Build history of the part. All positions in model axes, mm. A direction names the side the tool comes from. Round coordinates to 2 decimals unless told otherwise and drop trailing zeros. Loops run counter-clockwise (first coordinate to the right, second up) from the corner with the lowest first, then second, coordinate; pieces in that order, holes last. Notation, with made-up numbers: (79, 43) - (109, 43) arc R12 cw to (109, 61) - close; hole circle Ø6 at (-9, -5). An arc over 180 degrees is marked (long way). Use a Markdown table: item, result.
from build123d import *

# Parameters (mm, degrees)
SKETCH_1_W               = 56
SKETCH_1_H               = 14
F_56X14_3_3MM_DEPTH      = 3
SKETCH_2_W               = 40
SKETCH_2_H               = 11
CUT_EXTRUDE_40_4_3_DEPTH = 3
SKETCH_3_W               = 8
SKETCH_3_H               = 25
F_5_M2_5X10_DEPTH        = 5
SKETCH_4_R               = 1.55
CUT_EXTRUDE_3_1_48_DEPTH = 5
SKETCH_5_R               = 1.8
CUT_EXTRUDE_993_DEPTH    = 3


with BuildPart() as part:
    # 草图1 → 相机小底脚56x14_厚3_单向3mm (new body)
    with BuildSketch(Plane(origin=(0, 0, 0), x_dir=(1, 0, 0), z_dir=(0, 1, 0))):
        with Locations((0, 2)):
            Rectangle(SKETCH_1_W, SKETCH_1_H)
    extrude(amount=F_56X14_3_3MM_DEPTH)

    # 草图2 → 底脚中央40宽镂空_只留后横梁4_贯穿底脚3 (cut)
    with BuildSketch(Plane(origin=(0, 0, 0), x_dir=(1, 0, 0), z_dir=(0, 1, 0))):
        with Locations((0, -0.5)):
            Rectangle(SKETCH_2_W, SKETCH_2_H)
    extrude(amount=CUT_EXTRUDE_40_4_3_DEPTH, mode=Mode.SUBTRACT)

    # 草图3 → 双耳支撑臂厚5_沿用M2.5x10尺寸链 (add)
    with BuildSketch(Plane.XY):
        with Locations((-24, 15.5)):
            Rectangle(SKETCH_3_W, SKETCH_3_H)
        with Locations((24, 15.5)):
            Rectangle(SKETCH_3_W, SKETCH_3_H)
    extrude(amount=F_5_M2_5X10_DEPTH)

    # 草图4 → 双耳原孔3.1_孔距48_圆孔不加大_贯穿 (cut)
    with BuildSketch(Plane.XY):
        with Locations((-24, 24)):
            Circle(SKETCH_4_R)
        with Locations((24, 24)):
            Circle(SKETCH_4_R)
    extrude(amount=CUT_EXTRUDE_3_1_48_DEPTH, mode=Mode.SUBTRACT)

    # 草图5 → Cut-Extrude 993 (cut)
    with BuildSketch(Plane(origin=(0, 0, 0), x_dir=(1, 0, 0), z_dir=(0, 1, 0))):
        with Locations(Location((-24, 4.5, 0), (0, 0, 270))):
            Circle(SKETCH_5_R)
        with Locations(Location((24, 4.5, 0), (0, 0, 270))):
            Circle(SKETCH_5_R)
    extrude(amount=CUT_EXTRUDE_993_DEPTH, mode=Mode.SUBTRACT)


solid = part.part
Q1. Cut at D-D, the plane y = 6. List the corners of the cut face in (x, z), plus the area to 3 significant figures.
Results found:
| item | result |
|---|---|
| outline | (-28, 0) - (-20, 0) - (-20, 5) - (-28, 5) - close; (20, 0) - (28, 0) - (28, 5) - (20, 5) - close |
| area | 80.0 mm2 |
Q2. Pull direction X, two halves, no side cores. Call faces 4 (the face through (23.798, 25.537, 2.465)), 5 (the face through (28, 11, 1)), 6 (the face through (24, 14, 5)): pulls with the +X half, pulls with the -X half, needs draft (parallel to the pull), parting line crosses it, or undercut.
Results found:
| item | result |
|---|---|
| face 4 | undercut |
| face 5 | pulls with the +X half |
| face 6 | needs draft |
Q3. Drop flat-ended pins along their axis: pin 1 (5 mm diameter, centred on x = -18, z = 1, fed in from -Y); pin 2 (0.9 mm diameter, centred on x = 7, y = 1, fed in from +Z); pin 3 (3 mm diameter, centred on x = 24, z = -4.5, fed in from +Y); pin 4 (2.5 mm diameter, centred on x = -23.5, y = 9.5, fed in from -Z). Give the stop position or say it passes through.
Results found:
| item | result |
|---|---|
| pin 1 | stops at y = 0 |
| pin 2 | stops at z = -5 |
| pin 3 | passes through |
| pin 4 | stops at z = 0 |
Q4. Cut at A-A, the plane z = 2.75. List the corners of the cut face in (x, y), plus the area to 3 significant figures.
Results found:
| item | result |
|---|---|
| outline | (-28, 0) - (-20, 0) - (-20, 28) - (-28, 28) - close; (20, 0) - (28, 0) - (28, 28) - (20, 28) - close; hole circle Ø3.1 at (-24, 24); hole circle Ø3.1 at (24, 24) |
| area | 433 mm2 |
Q5. Which spindle directions (+Z, -Z, +X, -X, +Y, -Y) get a long thin tool onto all of the face, cutting with end or side? Do faces 1 (the face through (0, 3, -7)), 2 (the face through (25.518, 1.479, -3.532)), 3 (the face through (0, 1, -5)). Say none if no direction does.
Results found:
| item | result |
|---|---|
| face 1 | -Z, +X, -X, +Y |
| face 2 | +Y, -Y |
| face 3 | +Z, +Y, -Y |
Q6. Cut at B-B, the plane y = 24. List the corners of the cut face in (x, z).
Results found:
| item | result |
|---|---|
| outline | (-28, 0) - (-25.55, 0) - (-25.55, 5) - (-28, 5) - close; (-22.45, 0) - (-20, 0) - (-20, 5) - (-22.45, 5) - close; (20, 0) - (22.45, 0) - (22.45, 5) - (20, 5) - close; (25.55, 0) - (28, 0) - (28, 5) - (25.55, 5) - close |
Q7. Cut at C-C, the plane x = 24. List the corners of the cut face in (y, z).
Results found:
| item | result |
|---|---|
| outline | (0, -9) - (3, -9) - (3, -6.3) - (0, -6.3) - close; (0, -2.7) - (3, -2.7) - (3, 0) - (22.45, 0) - (22.45, 5) - (0, 5) - close; (25.55, 0) - (28, 0) - (28, 5) - (25.55, 5) - close |
Q8. Probe line 1 (X direction, y = 2.25, z = -4.5); line 2 (Y direction, x = -24, z = 3.75); line 3 (X direction, y = 5.75, z = 3.5). List the from-to ranges inside material, lowest first.
Results found:
| item | result |
|---|---|
| line 1 | x = -28 to -25.8, -22.2 to -20, 20 to 22.2, 25.8 to 28 |
| line 2 | y = 0 to 22.45, 25.55 to 28 |
| line 3 | x = -28 to -20, 20 to 28 |
